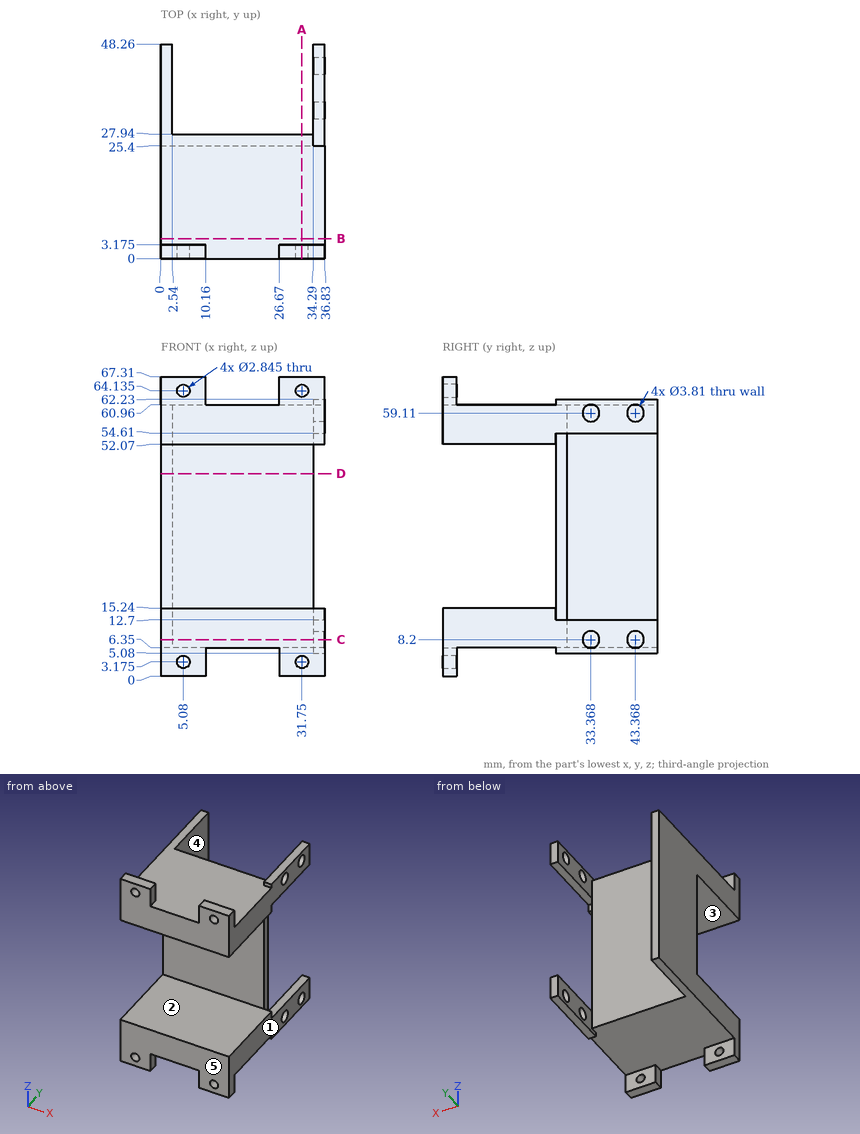
For this review, use the dimensioned drawing (mm, ordinates from the lowest corner) and the shaded views. A direction names the side the tool comes from. Give positions to 0.01 mm unless a question says otherwise; leave off trailing zeros. Order: outer loops, then holes, each group sorted by start corner. A loop starts at its lowest first (then second) coordinate and runs counter-clockwise, first axis right, second up.
1) Take a section at D-D (z = 45.5). Give the boundary of the cut face in (x, y), then the cut area to 3 significant figures.
2) The part is to be moulded in two halves that separate along Z. For the marked faces 1 and 2, say which applies: released by +Z, released by -Z, zero draft, split by the parting line, or undercut.
3) Wall thickness on line 1 (Y direction, x = 35, z = 59); line 2 (Z direction, x = 15, y = 6); line 3 (Y direction, x = 9, z = 17): over which ranges is each line inside the solid? List them lowest first.
4) For the marked faces 3, 4 and 5, list the 3-axis set-ups (+Z, -Z, +X, -X, +Y, -Y) from which the entire face can be reached by the end or side of a thin tool; tool diameter is ignored.
5) Take a section at A-A (x = 31.75). State how many separate pieces and enclosed holes the cut face has.
6) Take a section at B-B (y = 4.5). Give the boundary of the cut face in (x, z).
7) Insertion check: pin 1 (12 mm diameter, centred on x = 29, z = 26.5, fed in from -Y); pin 2 (4 mm diameter, centred on y = 32, z = 50, fed in from +X); pin 3 (4 mm diameter, centred on x = 16, z = 16, fed in from +Y). Each pin has a flat end and moves straight along its axis. Give the tip position at first contact, or say it passes through.
8) Take a section at C-C (z = 8.2). Give the boundary of the cut face in (x, y).
Derived:
1. outline: (0, 25.4) - (34.29, 25.4) - (34.29, 27.94) - (2.54, 27.94) - (2.54, 48.26) - (0, 48.26) - close
1. area: 139 mm2
2. face 1: zero draft
2. face 2: undercut
3. line 1: y = 0 to 31.47, 35.27 to 41.47, 45.27 to 48.26
3. line 2: z = 6.35 to 15.24, 52.07 to 60.96
3. line 3: y = 25.4 to 27.94
4. face 3: +X, -X, -Y
4. face 4: +Z, -Z, +Y
4. face 5: +Z, -Z, +X, -X, -Y
5. separate pieces: 3
5. enclosed holes: 0
6. outline: (0, 6.35) - (36.83, 6.35) - (36.83, 15.24) - (0, 15.24) - close; (0, 52.07) - (36.83, 52.07) - (36.83, 60.96) - (0, 60.96) - close
7. pin 1: stops at y = 25.4
7. pin 2: stops at x = 2.54
7. pin 3: stops at y = 27.94
8. outline: (0, 0) - (36.83, 0) - (36.83, 31.46) - (34.29, 31.46) - (34.29, 27.94) - (2.54, 27.94) - (2.54, 48.26) - (0, 48.26) - close; (34.29, 35.27) - (36.83, 35.27) - (36.83, 41.46) - (34.29, 41.46) - close; (34.29, 45.27) - (36.83, 45.27) - (36.83, 48.26) - (34.29, 48.26) - close
